For this review, use the dimensioned drawing (mm, ordinates from the lowest corner) and the shaded views. Round coordinates to 2 decimals unless told otherwise and drop trailing zeros. Order: outer loops, then holes, each group sorted by start corner. A loop starts at its lowest first (then second) coordinate and runs counter-clockwise, first axis right, second up. Notation, with made-up numbers: M 57,25.25 L 101,25.25 A24 ccw 101,63.25 Z; hole C 14,-23 d6. An arc over 180 degrees is marked long. Use a Markdown table: item, result. Add a question column.
1. Insertion check: P1, Ø6, axis at x = 26, z = 28.5, coming from the -Y side; P2, Ø1, axis at y = 69, z = 27, coming from the +X side (1 decimal); P3, Ø4, axis at y = 39.5, z = 7, coming from the +X side; P4, Ø3.5, axis at x = 30.5, z = 47.5, coming from the +Y side. Each pin has a flat end and moves straight along its axis. Give the tip position at first contact, or say it passes through.
2. Consider section A-A on z = 25. State the section outline as (x, y) points.
3. The part is to be moulded in two halves that separate along Z. For the marked faces 1, 2 and 3, say which applies: +Z half, -Z half, draft (parallel to the pull), parting line (faces both ways), or undercut.
4. Consider section B-B on y = 64.5. State the section outline as (x, z) points.
5. To check wall thickness, follow probe 1 along X at (y, z) = (71, 25); probe 2 along Y at (x, z) = (38, 35). State the ranges of each line that lie inside material, in increasing order.
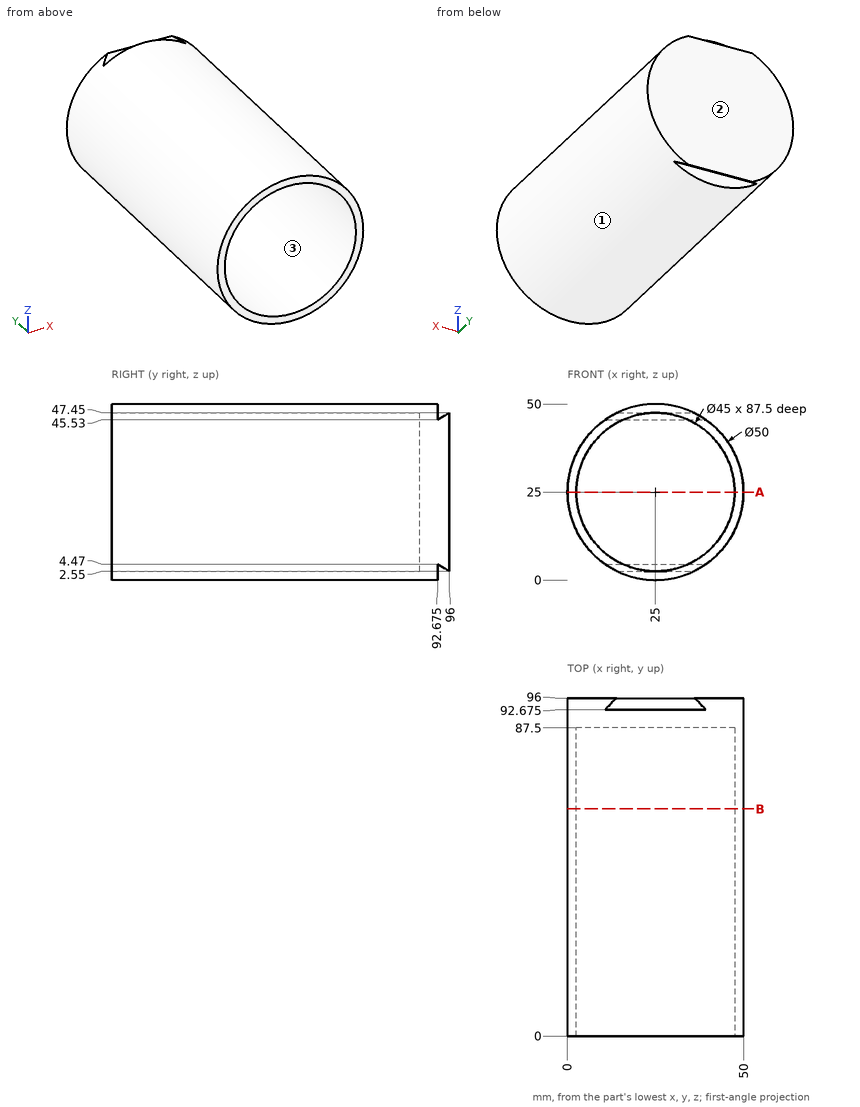
Answer block:
| question | item | result |
|---|---|---|
| 1 | P1 | y = 87.5 |
| 1 | P2 | x = 50 |
| 1 | P3 | x = 44.21 |
| 1 | P4 | y = 96 |
| 2 | outline | M 0,0 L 2.5,0 L 2.5,87.5 L 47.5,87.5 L 47.5,0 L 50,0 L 50,96 L 0,96 Z |
| 3 | face 1 | parting line |
| 3 | face 2 | draft |
| 3 | face 3 | undercut |
| 4 | outline | C 25,25 d50; hole C 25,25 d45 |
| 5 | probe 1 | 0 to 2.5, 47.5 to 50 |
| 5 | probe 2 | 87.5 to 96 |
